from build123d import *

# Parameters (mm, degrees)
CYLINDER005_R     = 3
CYLINDER005_DEPTH = 10
CYLINDER004_R     = 3
CYLINDER004_DEPTH = 10
CYLINDER003_R     = 3
CYLINDER003_DEPTH = 10
CYLINDER002_R     = 3
CYLINDER002_DEPTH = 10
CYLINDER001_R     = 47.5
CYLINDER001_DEPTH = 30
BOX_W             = 110
BOX_H             = 110
BOX_DEPTH         = 3
CYLINDER_R        = 49
CYLINDER_DEPTH    = 30


with BuildPart() as cylinder005:
    # Cylinder005 → Cylinder005 (new body)
    with BuildSketch(Plane(origin=(100.5, 9.5, 0), x_dir=(1, 0, 0), z_dir=(0, 0, 1))):
        Circle(CYLINDER005_R)
    extrude(amount=CYLINDER005_DEPTH)


with BuildPart() as cylinder004:
    # Cylinder004 → Cylinder004 (new body)
    with BuildSketch(Plane(origin=(100.5, 100.5, 0), x_dir=(1, 0, 0), z_dir=(0, 0, 1))):
        Circle(CYLINDER004_R)
    extrude(amount=CYLINDER004_DEPTH)


with BuildPart() as cylinder003:
    # Cylinder003 → Cylinder003 (new body)
    with BuildSketch(Plane(origin=(9.5, 100.5, 0), x_dir=(1, 0, 0), z_dir=(0, 0, 1))):
        Circle(CYLINDER003_R)
    extrude(amount=CYLINDER003_DEPTH)


with BuildPart() as cylinder002:
    # Cylinder002 → Cylinder002 (new body)
    with BuildSketch(Plane(origin=(9.5, 9.5, 0), x_dir=(1, 0, 0), z_dir=(0, 0, 1))):
        Circle(CYLINDER002_R)
    extrude(amount=CYLINDER002_DEPTH)


with BuildPart() as cylinder001:
    # Cylinder001 → Cylinder001 (new body)
    with BuildSketch(Plane(origin=(55, 55, 0), x_dir=(1, 0, 0), z_dir=(0, 0, 1))):
        Circle(CYLINDER001_R)
    extrude(amount=CYLINDER001_DEPTH)


with BuildPart() as cut:
    # Box → Box (new body)
    with BuildSketch(Plane.XY):
        with Locations((55, 55)):
            Rectangle(BOX_W, BOX_H)
    extrude(amount=BOX_DEPTH)

    # Cut: cut Cylinder001
    add(cylinder001.part, mode=Mode.SUBTRACT)


with BuildPart() as cut005:
    # Cylinder → Cylinder (new body)
    with BuildSketch(Plane(origin=(55, 55, 0), x_dir=(1, 0, 0), z_dir=(0, 0, 1))):
        Circle(CYLINDER_R)
    extrude(amount=CYLINDER_DEPTH)

    # Cut001: cut Cylinder001
    add(cylinder001.part, mode=Mode.SUBTRACT)

    # Fusion: union Cut
    add(cut.part)

    # Cut002: cut Cylinder002
    add(cylinder002.part, mode=Mode.SUBTRACT)

    # Cut003: cut Cylinder003
    add(cylinder003.part, mode=Mode.SUBTRACT)

    # Cut004: cut Cylinder004
    add(cylinder004.part, mode=Mode.SUBTRACT)

    # Cut005: cut Cylinder005
    add(cylinder005.part, mode=Mode.SUBTRACT)


solid = cut005.part
Can you work these out from the model? Positions are in its coordinate system, mm. A direction names the side the tool comes from. Coordinates: 2 decimals unless noted, no trailing zeros. Loops run counter-clockwise (first coordinate to the right, second up) from the corner with the lowest first, then second, coordinate; pieces in that order, holes last. Notation, with made-up numbers: M 84,-30 L 125,-30 A27 cw 125,4 Z; hole C -9,63 d10. An arc over 180 degrees is marked long. Return JSON: item names as keys, results as strings. Group by question number.
Item 1: Imagine slicing it at A-A (y = 55). Please give me the cut outline in (x, z), and give its area (3 significant figures).
Item 2: Thinking about a two-plate mould opening in Y: for faces 1 (the flat face through (110, 54, 1)), 2 (the cylindrical face through (12.27, 8.35, 1.48)), 3 (the cylindrical face through (100.264, 36.233, 16.311)), which applies, released by +Y, released by -Y, zero draft, split by the parting line, or undercut?
Item 3: Imagine slicing it at C-C (z = 14). Please give me the cut outline in (x, y), and give its area (3 significant figures).
Item 4: If I drill on L1, parallel to Y at x = 54.5, z = 16.25; L2, parallel to Z at x = 93, y = 101.5; L3, parallel to X at y = 25.5, z = 24, over which ranges is the centre line in solid material (lowest first)? Write a range as from..to.
Item 5: I'm going to push flat-ended pins straight in: pin 1 Ø2 at (x, z) = (82.5, 15.5) entering from -Y; pin 2 Ø3 at (y, z) = (49, 10) entering from +X; pin 3 Ø1 at (x, z) = (14, 26.5) entering from +Y. Where does each tip first touch, or does it pass through?
Item 6: On a 3-axis mill with a long thin cutter (end or side, diameter ignored), from which of +Z, -Z, +X, -X, +Y, -Y can I reach the whole of each face in a straight line? I mean faces 4 (the flat face through (54, 0, 1)), 5 (the flat face through (5, 56, 3)). Say none if no direction works.
Item 7: Imagine slicing it at D-D (y = 100.5). Please give me the cut outline in (x, z).
Verdict:
{
 "1": {"outline": "M 0,0 L 7.5,0 L 7.5,30 L 6,30 L 6,3 L 0,3 Z; M 102.5,0 L 110,0 L 110,3 L 104,3 L 104,30 L 102.5,30 Z", "area": "126 mm^2"},
 "2": {"face 1": "zero draft", "face 2": "undercut", "face 3": "split by the parting line"},
 "3": {"outline": "C 55,55 d98; hole C 55,55 d95", "area": "455 mm^2"},
 "4": {"L1": "y = 6..7.5, 102.5..104", "L2": "z = 0..3", "L3": "x = 15.88..17.77, 92.23..94.12"},
 "5": {"pin 1": "stops at y = 13.78", "pin 2": "stops at x = 103.79", "pin 3": "stops at y = 82.58"},
 "6": {"face 4": "+Z, -Z, +X, -X, -Y", "face 5": "+Z"},
 "7": {"outline": "M 0,0 L 6.5,0 L 6.5,3 L 0,3 Z; M 12.5,0 L 41.36,0 L 41.36,30 L 36.81,30 L 36.81,3 L 12.5,3 Z; M 68.64,0 L 97.5,0 L 97.5,3 L 73.19,3 L 73.19,30 L 68.64,30 Z; M 103.5,0 L 110,0 L 110,3 L 103.5,3 Z"}
}
